from build123d import *

# Parameters (mm, degrees)
BOSS_EXTRUDE1_DEPTH     = 76.2
CUT_EXTRUDE1_DEPTH      = 32
CUT_EXTRUDE1_DEPTH_BACK = 11.07899994
SKETCH2_W               = 46.228
SKETCH2_H               = 67.056
CHAMFER2_SIZE           = 11.313708499
CHAMFER2_SIZE_2         = 8
CHAMFER3_SIZE           = 10
CHAMFER3_SIZE2          = 7.071067812
SKETCH3_R               = 3.175
CUT_EXTRUDE2_DEPTH      = 89.533824561
SKETCH8_W               = 43.728932188
SKETCH8_H               = 9.525
BOSS_EXTRUDE3_DEPTH     = 25.4
SKETCH9_R               = 3.175
CUT_EXTRUDE3_DEPTH      = 70.342045029
FILLET2_R               = 6.35


with BuildPart() as part:
    # Sketch1 → Boss-Extrude1 (new body)
    with BuildSketch(Plane.XY):
        Polygon((30.841032184, 29.793919389), (-19.958967816, -21.006080611), (30.841032184, -21.006080611), align=None)
    extrude(amount=BOSS_EXTRUDE1_DEPTH)

    # Sketch2 → Cut-Extrude1 (cut, two sides: drawn at the far end of the back side and taken through both)
    with BuildSketch(Plane(origin=(0, 0, 0), x_dir=(1, 0, 0), z_dir=(0, 1, 0)).offset(-CUT_EXTRUDE1_DEPTH_BACK)):
        with Locations((3.155032184, -38.1)):
            Rectangle(SKETCH2_W, SKETCH2_H)
    extrude(amount=CUT_EXTRUDE1_DEPTH + CUT_EXTRUDE1_DEPTH_BACK, mode=Mode.SUBTRACT)

    # Chamfer2
    # the kernel refuses this chamfer: 11.313708499, 8 mm, written as the material it takes off along each edge
    with BuildSketch(Plane(origin=(30.841032184, 29.793919389, -29.095271678), x_dir=(-0.7262819568766876, -0.6873969152646594, 0), z_dir=(0, 0, 1))) as chamfer2_piece_1:
        Polygon((CHAMFER2_SIZE * 0.99962191691, CHAMFER2_SIZE * 0.0274958766105), (CHAMFER2_SIZE_2 * 0.687396915265, CHAMFER2_SIZE_2 * 0.726281956877), (0, 0), align=None)
    extrude(amount=134.390543355, mode=Mode.SUBTRACT)

    # Chamfer3
    chamfer3_edges = [part.edges().sort_by_distance(p)[0] for p in [
        (-19.958967816, -21.006080611, 38.1),
    ]]
    chamfer3_side = [part.faces().sort_by_distance(p)[0] for p in [
        (1.441032184, 0.393919389, 0.973145416),
    ]]
    chamfer(chamfer3_edges, length=CHAMFER3_SIZE, length2=CHAMFER3_SIZE2, reference=chamfer3_side[0])

    # Sketch3 → Cut-Extrude2 (cut, through all)
    with BuildSketch(Plane(origin=(0, -11.07899994, 0), x_dir=(1, 0, 0), z_dir=(0, 1, 0))):
        with Locations(Location((8.97656609, -12.7, 0), (0, 0, 270))):
            Circle(SKETCH3_R)
    extrude(amount=-CUT_EXTRUDE2_DEPTH, mode=Mode.SUBTRACT)

    # Sketch8 → Boss-Extrude3 (add)
    with BuildSketch(Plane.XZ.offset(21.006080611)):
        with Locations((8.97656609, 30.1625)):
            Rectangle(SKETCH8_W, SKETCH8_H)
    extrude(amount=BOSS_EXTRUDE3_DEPTH)

    # Sketch9 → Cut-Extrude3 (cut, through all)
    with BuildSketch(Plane.XY.offset(34.925)):
        with Locations((8.97656609, -33.706080611)):
            Circle(SKETCH9_R)
    extrude(amount=-CUT_EXTRUDE3_DEPTH, mode=Mode.SUBTRACT)

    # Fillet2
    fillet2_edges = [part.edges().sort_by_distance(p)[0] for p in [
        (8.97656609, -21.006080611, 34.925),
        (8.97656609, -21.006080611, 25.4),
    ]]
    fillet(fillet2_edges, radius=FILLET2_R)


solid = part.part
Could you check a few things on this model? Use its own coordinates, in mm. A direction names the side the tool comes from. Give positions to 0.01 mm unless a question says otherwise; leave off trailing zeros. Order: outer loops, then holes, each group sorted by start corner. A loop starts at its lowest first (then second) coordinate and runs counter-clockwise, first axis right, second up. Notation, with made-up numbers: (33, 75) - (50, 75) arc R22 cw to (50, 90) - close; hole circle Ø2 at (-15.75, -15). An arc over 180 degrees is marked (long way). One line per item, written item: value. Start each with the question number.
1. Imagine slicing it at B-B on x = 1. List the corners of the cut face in (y, z) for me (3 decimals).
2. Thinking about a two-plate mould opening in Z: for faces 1 (the face through (9, -21.006, 9)), 2 (the face through (14, -4, 76.2)), 3 (the face through (12, 1, 4.572)), which applies, +Z half, -Z half, draft (parallel to the pull), parting line (faces both ways), or undercut?
3. Imagine slicing it at A-A on z = 12.7. List the corners of the cut face in (x, y) for me, plus the area to 3 significant figures.
4. Imagine slicing it at C-C on z = 59. List the corners of the cut face in (x, y) for me.
5. For faces 4 (the face through (9, -46.406, 30)), 5 (the face through (30.841, -5, 38)), 6 (the face through (8, -11.079, 38)), 7 (the face through (9, -39, 25.4)), 8 (the face through (9, -39, 34.925)), which set-ups out of +Z, -Z, +X, -X, +Y, -Y let a thin tool reach every point of the face, with its end or its side?
6. Imagine slicing it at D-D on y = -42. List the corners of the cut face in (x, z) for me (3 decimals), plus the area to 3 significant figures.
7. For P1, Ø8.5, axis at x = 8.98, y = -33.71, coming from the -Z side; P2, Ø3, axis at x = -3, y = -31, coming from the +Z side (3 decimals); P3, Ø8, axis at y = -29.5, z = 37, coming from the +X side; P4, Ø16.5, axis at y = 7.5, z = 33, coming from the -X side, each with a flat end and sliding along its axis, tell me the tip position at first contact or that it passes through.
8. If I drill on probe 1 along Z at (x, y) = (23.5, 2); probe 2 along X at (y, z) = (-16.5, 12.7); probe 3 along Y at (x, z) = (-4, 52.5), over which ranges is the centre line in solid material (lowest first)?
Values:
1. outline: (-46.406, 25.4) - (-27.356, 25.4) arc R6.35 cw to (-21.006, 19.05) - (-21.006, 0) - (-0.047, 0) - (-0.047, 4.572) - (-11.079, 4.572) - (-11.079, 71.628) - (-0.047, 71.628) - (-0.047, 76.2) - (-21.006, 76.2) - (-21.006, 41.275) arc R6.35 cw to (-27.356, 34.925) - (-46.406, 34.925) - close
2. face 1: draft
2. face 2: +Z half
2. face 3: undercut
3. outline: (-12.89, -21.01) - (5.8, -21.01) - (5.8, -11.08) - (-10.03, -11.08) - (-12.89, -13.94) - close; (12.15, -21.01) - (30.84, -21.01) - (30.84, 21.79) - (26.27, 21.79) - (26.27, -11.08) - (12.15, -11.08) - close
3. area: 517 mm²
4. outline: (-12.89, -21.01) - (30.84, -21.01) - (30.84, 21.79) - (26.27, 21.79) - (26.27, -11.08) - (-10.03, -11.08) - (-12.89, -13.94) - close
5. face 4: +Z, -Z, +X, -X, -Y
5. face 5: +Z, -Z, +X, +Y, -Y
5. face 6: -X, +Y
5. face 7: -Z, +X, -X, -Y
5. face 8: +Z, +X, -X, -Y
6. outline: (-12.888, 25.4) - (30.841, 25.4) - (30.841, 34.925) - (-12.888, 34.925) - close
6. area: 417 mm²
7. P1: z = 25.4
7. P2: z = 34.925
7. P3: x = 30.84
7. P4: x = 26.27
8. probe 1: 0 to 4.57, 71.63 to 76.2
8. probe 2: -12.89 to 5.8, 12.15 to 30.84
8. probe 3: -21.01 to -11.08
